Verification items for this drawing (mm, ordinates from the low corner). A direction names the side the tool comes from. Give positions to 0.01 mm unless a question says otherwise; leave off trailing zeros. Loops run counter-clockwise (first coordinate to the right, second up) from the corner with the lowest first, then second, coordinate; pieces in that order, holes last. Notation, with made-up numbers: (84, -22) -> (118, -22) arc R15 cw to (118, -8) -> close; hole circle Ø8 at (-18, -10). An arc over 180 degrees is marked (long way). Answer as a JSON object with one key per item and string values.
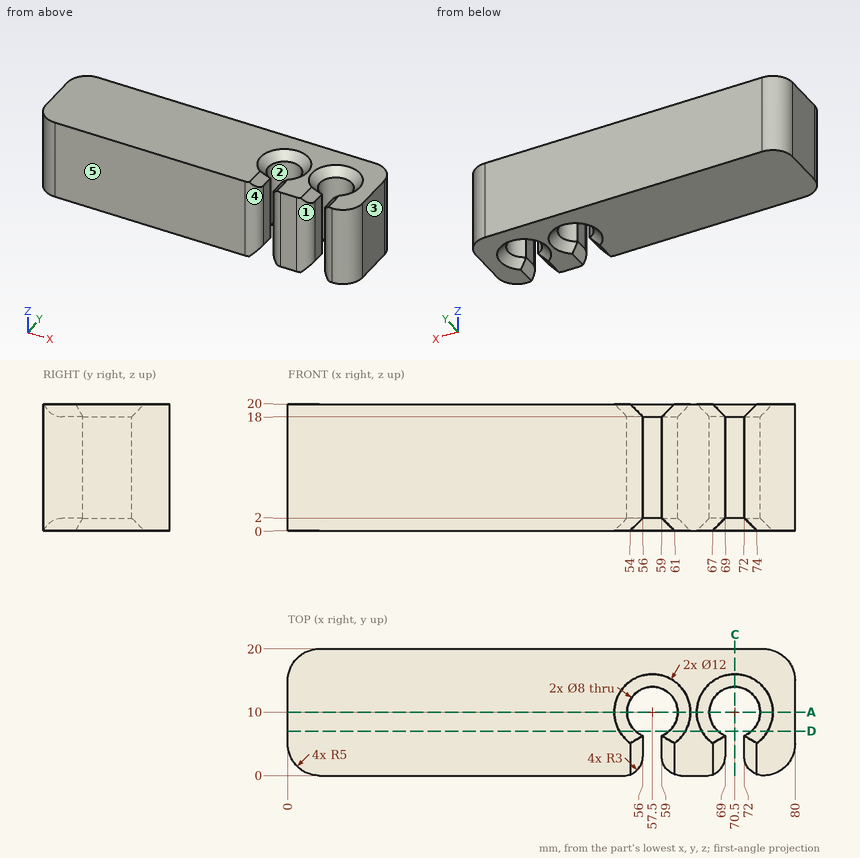
1) Section check C-C on x = 70.5. Record the cut outline in (y, z), plus the area to 3 significant figures.
Geometry check:
{"outline": "(14, 2) -> (16, 0) -> (20, 0) -> (20, 20) -> (16, 20) -> (14, 18) -> close", "area": "116 mm2"}
2) Depth check by flat-ended pin: P1, Ø1.6, axis at y = 4, z = 6, coming from the +X side; P2, Ø6.5, axis at x = 70.5, y = 10, coming from the -Z side; P3, Ø1.6, axis at y = 4, z = 13, coming from the -X side; P4, Ø9, axis at x = 57.5, y = 10, coming from the -Z side. Enter the tip coordinate at first touch or a pass-through.
Geometry check:
{"P1": "stops at x = 80", "P2": "passes through", "P3": "stops at x = 0", "P4": "stops at z = 1.5"}
3) Draft check along X on the marked faces 3, 4 and 5. Enter one of: pulls with the +X half, pulls with the -X half, needs draft (parallel to the pull), parting line crosses it, or undercut.
Geometry check:
{"face 3": "pulls with the +X half", "face 4": "undercut", "face 5": "needs draft"}
4) Section check A-A on y = 10. Record the cut outline in (x, z).
Geometry check:
{"outline": "(0, 0) -> (51.5, 0) -> (53.5, 2) -> (53.5, 18) -> (51.5, 20) -> (0, 20) -> close; (61.5, 2) -> (63.5, 0) -> (64.5, 0) -> (66.5, 2) -> (66.5, 18) -> (64.5, 20) -> (63.5, 20) -> (61.5, 18) -> close; (74.5, 2) -> (76.5, 0) -> (80, 0) -> (80, 20) -> (76.5, 20) -> (74.5, 18) -> close"}
5) Material ranges on line 1 along X through (y, z) = (5.25, 2.5); line 2 along X through (y, z) = (10, 10); line 3 along Y through (x, z) = (70.5, 14.75), recorded low to high. Write a range as from..to.
Geometry check:
{"line 1": "x = 0..56, 59..69, 72..80", "line 2": "x = 0..53.5, 61.5..66.5, 74.5..80", "line 3": "y = 14..20"}
6) Section check D-D on y = 7. Count the separate pieces of the cut face and the enclosed holes in it, plus the area to 3 significant figures.
Geometry check:
{"separate pieces": "3", "enclosed holes": "0", "area": "1,370 mm2"}
7) Tool access check on the marked faces 1 and 2. Record the directions out of +Z, -Z, +X, -X, +Y, -Y that give a thin tool (end or side, any length) a straight path to the whole face; none if there is none.
Geometry check:
{"face 1": "+Z, -Z, -Y", "face 2": "+Z, -Z"}
